from build123d import *

# Parameters (mm, degrees)
SKETCH1_W           = 43
SKETCH1_H           = 225
SKETCH2_R           = 23.5
BOSS_EXTRUDE1_DEPTH = 32
CIRPATTERN1_COUNT   = 3
SKETCH3_R           = 23.5
BOSS_EXTRUDE2_DEPTH = 32
CIRPATTERN2_COUNT   = 3
BOSS_EXTRUDE4_START = 20
SKETCH5_R           = 100
BOSS_EXTRUDE4_DEPTH = 62
SKETCH6_R           = 50
CUT_EXTRUDE2_DEPTH  = 25
SKETCH4_R           = 28
CUT_EXTRUDE1_DEPTH  = 342
SKETCH7_R           = 12
CUT_EXTRUDE3_DEPTH  = 15
CIRPATTERN3_COUNT   = 3


with BuildPart() as part:
    # Sketch1 → Revolve1 (revolve)
    with BuildSketch(Plane.XY):
        with Locations((118.5, 112.5)):
            Rectangle(SKETCH1_W, SKETCH1_H)
    revolve(axis=Axis((0, 0, 0), (0, 1, 0)))

    # Sketch2 → Boss-Extrude1 (add)
    with BuildSketch(Plane(origin=(0, 225, 0), x_dir=(1, 0, 0), z_dir=(0, 1, 0))):
        with BuildLine():
            ThreePointArc((50, 175), (0, 225), (-50, 175))
            Line((-50, 175), (-50, 130.766968306))
            ThreePointArc((-50, 130.766968306), (0, 140), (50, 130.766968306))
            Line((50, 130.766968306), (50, 175))
        make_face()
        with Locations((0, 175)):
            Circle(SKETCH2_R, mode=Mode.SUBTRACT)
    boss_extrude1 = extrude(amount=-BOSS_EXTRUDE1_DEPTH)

    # CirPattern1: Boss-Extrude1 ×3 about axis
    cirpattern1_axis = Axis((0, 0, 0), (0, 1, 0))
    for i in range(1, CIRPATTERN1_COUNT):
        add(boss_extrude1.rotate(cirpattern1_axis, i * 360 / CIRPATTERN1_COUNT))

    # Sketch3 → Boss-Extrude2 (add)
    with BuildSketch(Plane(origin=(0, 0, 0), x_dir=(1, 0, 0), z_dir=(0, 1, 0))):
        with BuildLine():
            ThreePointArc((50, 175), (0, 225), (-50, 175))
            Line((-50, 175), (-50, 130.766968306))
            ThreePointArc((-50, 130.766968306), (0, 140), (50, 130.766968306))
            Line((50, 130.766968306), (50, 175))
        make_face()
        with Locations((0, 175)):
            Circle(SKETCH3_R, mode=Mode.SUBTRACT)
    boss_extrude2 = extrude(amount=BOSS_EXTRUDE2_DEPTH)

    # CirPattern2: Boss-Extrude2 ×3 about axis
    cirpattern2_axis = Axis((0, 0, 0), (0, 1, 0))
    for i in range(1, CIRPATTERN2_COUNT):
        add(boss_extrude2.rotate(cirpattern2_axis, i * 360 / CIRPATTERN2_COUNT))

    # Sketch5 → Boss-Extrude4 (add)
    with BuildSketch(Plane.XY.offset(140).offset(BOSS_EXTRUDE4_START)):
        with Locations((0, 112.5)):
            Circle(SKETCH5_R)
    extrude(amount=-BOSS_EXTRUDE4_DEPTH)

    # Sketch6 → Cut-Extrude2 (cut)
    with BuildSketch(Plane.XY.offset(160)):
        with Locations((0, 112.5)):
            Circle(SKETCH6_R)
    extrude(amount=-CUT_EXTRUDE2_DEPTH, mode=Mode.SUBTRACT)

    # Sketch4 → Cut-Extrude1 (cut)
    with BuildSketch(Plane.XY.offset(140)):
        with Locations((0, 112.5)):
            Circle(SKETCH4_R)
    extrude(amount=-CUT_EXTRUDE1_DEPTH, mode=Mode.SUBTRACT)

    # Sketch7 → Cut-Extrude3 (cut)
    with BuildSketch(Plane.XY.offset(160)):
        with Locations((0, 188.646045953)):
            Circle(SKETCH7_R)
    cut_extrude3 = extrude(amount=-CUT_EXTRUDE3_DEPTH, mode=Mode.SUBTRACT)

    # CirPattern3: Cut-Extrude3 ×3 about axis
    cirpattern3_axis = Axis((0, 112.5, 0), (0, 0, 1))
    for i in range(1, CIRPATTERN3_COUNT):
        add(cut_extrude3.rotate(cirpattern3_axis, i * 360 / CIRPATTERN3_COUNT), mode=Mode.SUBTRACT)


solid = part.part
Verification items for the finished model (mm, model axes). A direction names the side the tool comes from. Coordinates: 2 decimals unless noted, no trailing zeros. Order: outer loops, then holes, each group sorted by start corner. A loop starts at its lowest first (then second) coordinate and runs counter-clockwise, first axis right, second up. Notation, with made-up numbers: M 25.5,-22 L 48.5,-22 A19 cw 48.5,-3 Z; hole C 33.25,4 d8. An arc over 180 degrees is marked long. One line per item, written item: value. Start each with the question number.
Item 1: Sectioned sample at C-C on y = 132. Record the cut outline in (x, z), then the cut area to 3 significant figures.
Item 2: Access from +Z, -Z, +X, -X, +Y, -Y to the whole of each face (thin tool, end or side, straight path). Record for faces 4 (the flat face through (0, 189, 145)), 5 (the flat face through (-50, 16, -153)), 6 (the flat face through (-107.67, 15.78, 119.9)).
Item 3: Depth check by flat-ended pin: P1, Ø4, axis at x = -110.5, y = 43.5, coming from the +Z side; P2, Ø1, axis at y = 101.5, z = 38, coming from the -X side; P3, Ø1.5, axis at y = 108, z = -34, coming from the -X side. Enter the tip coordinate at first touch or a pass-through.
Item 4: Mould release check, pull along Y, two halves, no side actions. Record for faces 1 (the cylindrical face through (77.03, 69.83, 152.6)), 2 (the flat face through (66, 74, 145)), 3 (the flat face through (107.133, 15.776, 119.588)): pulls with the +Y half, pulls with the -Y half, needs draft (parallel to the pull), parting line crosses it, or undercut.
Item 5: Sectioned sample at B-B on z = 87.5. Give the number of separate pieces and of enclosed holes in the cut face, then the cut area to 3 significant figures.
Item 6: Thickness scan on probe 1 along Y at (x, z) = (0, 150.75); probe 2 along Y at (x, z) = (-161, 117); probe 3 along Z at (x, y) = (0, 10). Record the ranges inside material, lowest first.
Item 7: Sectioned sample at A-A on z = 0. Record the cut outline in (x, y), then the cut area to 4 significant figures.
Calculated:
1. outline: M -98.08,99.9 A140 ccw -20.09,-138.55 L -20.09,-94.9 A97 cw -20.09,94.9 L -20.09,135 L -46.04,135 L -46.04,160 L -98.08,160 Z; M 20.09,-138.55 A140 ccw 98.08,99.9 L 98.08,160 L 46.04,160 L 46.04,135 L 20.09,135 L 20.09,94.9 A97 cw 20.09,-94.9 Z
1. area: 32,800 mm^2
2. face 4: +Z
2. face 5: -Z, -X, +Y, -Y
2. face 6: +Z, -Y
3. P1: z = 88.47
3. P2: x = -134.88
3. P3: x = -135.99
4. face 1: undercut
4. face 2: undercut
4. face 3: needs draft
5. separate pieces: 6
5. enclosed holes: 0
5. area: 36,100 mm^2
6. probe 1: 12.5 to 62.5, 162.5 to 176.65, 200.65 to 212.5
6. probe 2: 0 to 32, 193 to 225
6. probe 3: -225 to -198.5, -151.5 to -97, 97 to 140
7. outline: M -140,0 L -97,0 L -97,225 L -140,225 Z; M 97,0 L 140,0 L 140,225 L 97,225 Z
7. area: 19,350 mm^2
